Verification items for the finished model (mm, model axes). A direction names the side the tool comes from. Round coordinates to 2 decimals unless told otherwise and drop trailing zeros. Write each loop counter-clockwise with the first axis right and the second up, starting at its lowest first coordinate (ties: lowest second). Pieces come first, ordered by that corner, then holes. Notation, with made-up numbers: (81, 89) -> (114, 89) arc R7 cw to (114, 99) -> close; hole circle Ø11 at (59.25, 0.5). An arc over 180 degrees is marked (long way). Use CSV: the item, a comma, the result in double quotes.
```python
from build123d import *

# Parameters (mm, degrees)
F0_R     = 50
F1_DEPTH = 20
F2_R     = 47.5
F3_DEPTH = 120
F4_R     = 10
F5_SIZE  = 2.49999
F7_DEPTH = 13
F8_R     = 2
F9_DEPTH = 5


# Not quite as in the source:
# - a fillet or chamfer is up to 0.001 mm smaller than in the source, because OpenCascade refuses the exact size


with BuildPart() as f1:
    # F0 (on Top) → F1 (new body)
    with BuildSketch(Plane.XY):
        Circle(F0_R)
    extrude(amount=F1_DEPTH)

    # F2 (on face) → F3 (join)
    with BuildSketch(Plane.XY.offset(20)):
        Circle(F2_R)
    extrude(amount=F3_DEPTH)

    # F4
    f4_edges = [f1.edges().sort_by_distance(p)[0] for p in [
        (-47.5, 0, 140),
    ]]
    fillet(f4_edges, radius=F4_R)

    # F5 (size 2.5 in the source; OpenCascade refuses exactly that, so slightly less here)
    f5_edges = [f1.edges().sort_by_distance(p)[0] for p in [
        (-50, 0, 20),
    ]]
    chamfer(f5_edges, length=F5_SIZE)

    # F6 (on face) → F7 (join)
    with BuildSketch(Plane(origin=(0, 0, 0), x_dir=(1, 0, 0), z_dir=(0, 0, -1))):
        with BuildLine():
            Line((-50, 0), (-55, 0))
            Line((-55, 0), (-55, -5))
            Line((-55, -5), (-49.7493718553, -5))
            ThreePointArc((-49.7493718553, -5), (-49.9373036555, -2.503138753), (-50, 0))
        make_face()
        with BuildLine():
            Line((-55, 5), (-55, 0))
            Line((-55, 0), (-50, 0))
            ThreePointArc((-50, 0), (-49.9373036555, 2.503138753), (-49.7493718553, 5))
            Line((-49.7493718553, 5), (-55, 5))
        make_face()
    extrude(amount=-F7_DEPTH)

    # F8 (on face) → F9 (join)
    with BuildSketch(Plane(origin=(-55, 0, 0), x_dir=(0, -1, 0), z_dir=(-1, 0, 0))):
        with Locations((0, 6.5)):
            Circle(F8_R)
    extrude(amount=F9_DEPTH)


solid = f1.part
```
Q1. Access from +Z, -Z, +X, -X, +Y, -Y to the whole of each face (thin tool, end or side, straight path). Record for faces 1 (the cylindrical face through (-10.3, -46.37, 74.23)), 2 (the flat face through (-52, 5, 6)), 3 (the flat face through (-55, 2.2, 6.4)), 4 (the flat face through (-52, -5, 6)).
Filled in:
face 1,"+Z"
face 2,"+Z, -Z, -X, +Y"
face 3,"-X"
face 4,"+Z, -Z, -X, -Y"
Q2. Section check D-D (z = 118.5). Record the cut outline in (x, y), plus the area to 3 significant figures.
Filled in:
outline,"circle Ø95 at (0, 0)"
area,"7,090 mm²"
Q3. Material ranges on L1, parallel to X at y = -30, z = 19.5; L2, parallel to X at y = 35.5, z = 16; L3, parallel to Y at x = -0.5, z = 49.5, recorded low to high.
Filled in:
L1,"-37.47 to 37.47"
L2,"-35.21 to 35.21"
L3,"-47.5 to 47.5"
Q4. Section check A-A (z = 6.5). Record the cut outline in (x, y), plus the area to 3 significant figures.
Filled in:
outline,"(-60, -2) -> (-55, -2) -> (-55, -5) -> (-49.75, -5) arc R50 ccw (long way) to (-49.75, 5) -> (-55, 5) -> (-55, 2) -> (-60, 2) -> close"
area,"7,920 mm²"
Q5. Go/stop test with flat-tipped pins: P1, Ø3, axis at x = -48, y = -16.5, coming from the +Z side; P2, Ø10, axis at y = 36, z = 53.5, coming from the -X side; P3, Ø1, axis at y = 30, z = 20, coming from the -X side. Record where each tip stops, or that it passes through.
Filled in:
P1,"z = 18.24"
P2,"x = -35.99"
P3,"x = -37.58"
